from build123d import *

# Parameters (mm, degrees)
SKICA1_W                 = 55.6
SKICA1_H                 = 55.6
P_IDAT_VYSUNUT_M2_DEPTH  = 3
SKICA5_W                 = 5
SKICA5_H                 = 55.6
SKICA5_W_2               = 55.6
SKICA5_H_2               = 5
ODEBRAT_VYSUNUT_M3_DEPTH = 1
SKICA14_W                = 53.6
SKICA14_H                = 1.5
P_IDAT_VYSUNUT_M9_DEPTH  = 9.5
SKICA17_R                = 2
ODEBRAT_VYSUNUT_M8_DEPTH = 4
SKICA19_W                = 6.8
SKICA19_H                = 6.8
P_IDAT_VYSUNUT_M10_DEPTH = 12.5
SKICA20_R                = 2.4
ODEBRAT_VYSUNUT_M9_DEPTH = 1.7
ZAOBLIT1_R               = 2.5


with BuildPart() as part:
    # Skica1 → Přidat vysunutím2 (new body)
    with BuildSketch(Plane.XY):
        Rectangle(SKICA1_W, SKICA1_H)
    extrude(amount=P_IDAT_VYSUNUT_M2_DEPTH)

    # Skica5 → Odebrat vysunutím3 (cut)
    with BuildSketch(Plane(origin=(0, 0, 0), x_dir=(-1, 0, 0), z_dir=(0, 0, -1))):
        Rectangle(SKICA5_W, SKICA5_H)
        Rectangle(SKICA5_W_2, SKICA5_H_2)
    extrude(amount=-ODEBRAT_VYSUNUT_M3_DEPTH, mode=Mode.SUBTRACT)

    # Skica14 → Přidat vysunutím9 (add)
    with BuildSketch(Plane.XY.offset(3)):
        Polygon((27.8, 27.8), (-27.8, 27.8), (-27.8, -27.8), (-26.8, -27.8), (-26.8, -26.8), (-26.8, -26.3), (-26.8, 26.8), (26.8, 26.8), (26.8, -26.3), (26.8, -27.8), (27.8, -27.8), align=None)
        with Locations((0, -27.05)):
            Rectangle(SKICA14_W, SKICA14_H)
    extrude(amount=P_IDAT_VYSUNUT_M9_DEPTH)

    # Skica17 → Odebrat vysunutím8 (cut)
    with BuildSketch(Plane(origin=(0, 0, 1), x_dir=(-1, 0, 0), z_dir=(0, 0, -1))):
        with Locations((20.8, 0)):
            Circle(SKICA17_R)
        with Locations((-20.8, 0)):
            Circle(SKICA17_R)
        with Locations((0, 20.8)):
            Circle(SKICA17_R)
        with Locations((0, -20.8)):
            Circle(SKICA17_R)
    extrude(amount=-ODEBRAT_VYSUNUT_M8_DEPTH, mode=Mode.SUBTRACT)

    # Skica19 → Přidat vysunutím10 (add)
    with BuildSketch(Plane(origin=(0, 0, 0), x_dir=(-1, 0, 0), z_dir=(0, 0, -1))):
        with Locations((-24.4, 24.4)):
            Rectangle(SKICA19_W, SKICA19_H)
        with Locations((24.4, 24.4)):
            Rectangle(SKICA19_W, SKICA19_H)
        with Locations((-24.4, -24.4)):
            Rectangle(SKICA19_W, SKICA19_H)
        with Locations((24.4, -24.4)):
            Rectangle(SKICA19_W, SKICA19_H)
    extrude(amount=-P_IDAT_VYSUNUT_M10_DEPTH)

    # Skica20 → Odebrat vysunutím9 (cut)
    with BuildSketch(Plane.XY.offset(12.5)):
        with Locations((-23.9, -23.9)):
            Circle(SKICA20_R)
        with Locations((-23.9, 23.9)):
            Circle(SKICA20_R)
        with Locations((23.900280565, 23.9)):
            Circle(SKICA20_R)
        with Locations((23.900280565, -23.9)):
            Circle(SKICA20_R)
    extrude(amount=-ODEBRAT_VYSUNUT_M9_DEPTH, mode=Mode.SUBTRACT)

    # Zaoblit1
    zaoblit1_edges = [part.edges().sort_by_distance(p)[0] for p in [
        (21, 21, 7.75),
        (-21, 21, 7.75),
        (21, -21, 7.75),
        (-21, -21, 7.75),
    ]]
    fillet(zaoblit1_edges, radius=ZAOBLIT1_R)


solid = part.part
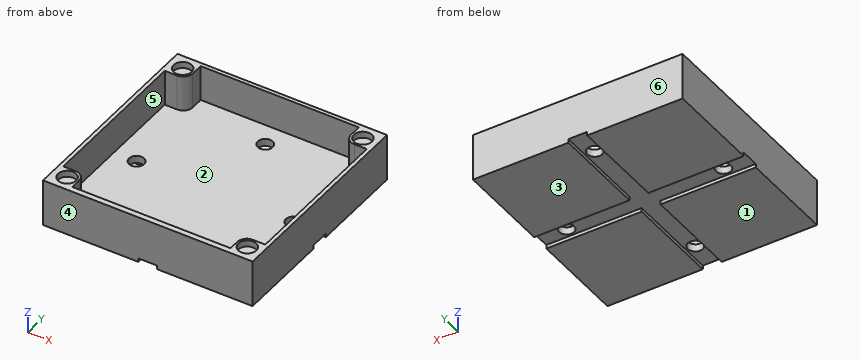
The model under review builds one solid part; all positions refer to its coordinate system, in mm. Face numbers are marked on the shaded views. A direction names the side the tool comes from. Round coordinates to 2 decimals unless told otherwise and drop trailing zeros. Order: outer loops, then holes, each group sorted by start corner. A loop starts at its lowest first (then second) coordinate and runs counter-clockwise, first axis right, second up. Notation, with made-up numbers: (-11, 82.25) -> (26, 82.25) arc R20 ccw to (26, 100.25) -> close; hole circle Ø6 at (-39, 5). An arc over 180 degrees is marked (long way). Write item = value, one per line. Start each with the question number.
Item 1: For line 1 along Y through (x, z) = (-23.9, 11.4); line 2 along Y through (x, z) = (0, 2.4); line 3 along X through (y, z) = (-6.5, 10), list the stretches that pass through material, from the lowest coordinate up.
Item 2: For the marked faces 1 and 2, list the 3-axis set-ups (+Z, -Z, +X, -X, +Y, -Y) from which the entire face can be reached by the end or side of a thin tool; tool diameter is ignored.
Item 3: Mouldability with a two-part tool opening along Y and no side actions: class the marked faces 3, 4, 5 and 6 as released by +Y, released by -Y, zero draft, split by the parting line, or undercut.
Item 4: Consider section A-A on x = 0. Write out the cut boundary in (y, z).
Item 5: Clearance check with flat-ended pins moving along their axes: pin 1 Ø3.5 at (x, y) = (0, 20.8) entering from +Z; pin 2 Ø4 at (x, y) = (17.5, 8.5) entering from +Z. State where each tip first meets the part, or that it passes through.
Item 6: Consider section C-C on y = -12. Write out the cut boundary in (x, z).
Item 7: Consider section B-B on z = 9.5. Write out the cut boundary in (x, y), plus the area to 3 significant figures.
Conclusion:
q1.line_1 = -27.8 to -26.3, -21.5 to -21, 21 to 21.5, 26.3 to 27.8
q1.line_2 = -27.8 to -22.8, -18.8 to 18.8, 22.8 to 27.8
q1.line_3 = -27.8 to -26.8, 26.8 to 27.8
q2.face_1 = -Z, +X, -X, +Y, -Y
q2.face_2 = +Z
q3.face_3 = zero draft
q3.face_4 = released by -Y
q3.face_5 = undercut
q3.face_6 = released by +Y
q4.outline = (-27.8, 1) -> (-22.8, 1) -> (-22.8, 3) -> (-26.3, 3) -> (-26.3, 12.5) -> (-27.8, 12.5) -> close; (-18.8, 1) -> (18.8, 1) -> (18.8, 3) -> (-18.8, 3) -> close; (22.8, 1) -> (27.8, 1) -> (27.8, 12.5) -> (26.8, 12.5) -> (26.8, 3) -> (22.8, 3) -> close
q5.pin_1 = through
q5.pin_2 = 3
q6.outline = (-27.8, 0) -> (-2.5, 0) -> (-2.5, 1) -> (2.5, 1) -> (2.5, 0) -> (27.8, 0) -> (27.8, 12.5) -> (26.8, 12.5) -> (26.8, 3) -> (-26.8, 3) -> (-26.8, 12.5) -> (-27.8, 12.5) -> close
q7.outline = (-27.8, -27.8) -> (27.8, -27.8) -> (27.8, 27.8) -> (-27.8, 27.8) -> close; hole (-26.8, -21) -> (-23.5, -21) arc R2.5 cw to (-21, -23.5) -> (-21, -26.3) -> (21, -26.3) -> (21, -23.5) arc R2.5 cw to (23.5, -21) -> (26.8, -21) -> (26.8, 21) -> (23.5, 21) arc R2.5 cw to (21, 23.5) -> (21, 26.8) -> (-21, 26.8) -> (-21, 23.5) arc R2.5 cw to (-23.5, 21) -> (-26.8, 21) -> close
q7.area = 369 mm2
